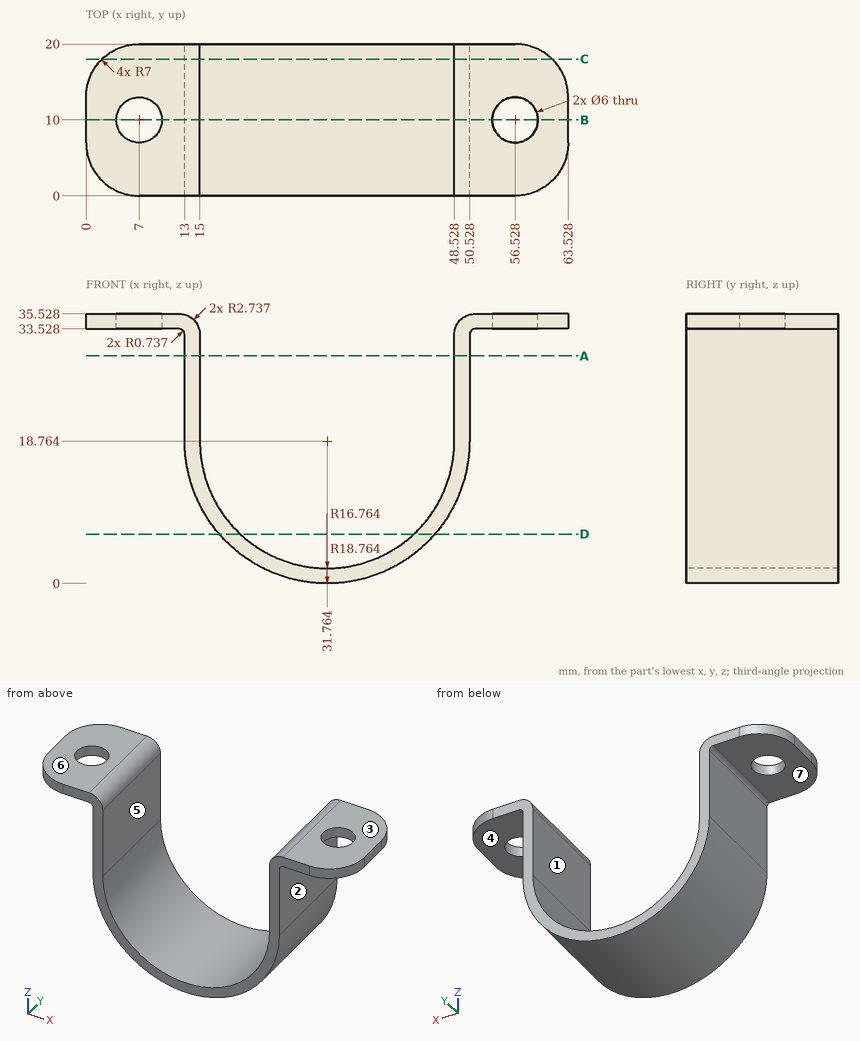
Part print with two shaded views. Sizes in mm from the minimum x, y, z corner. A direction names the side the tool comes from. Give positions to 0.01 mm unless a question says otherwise; leave off trailing zeros. Order: outer loops, then holes, each group sorted by start corner. A loop starts at its lowest first (then second) coordinate and runs counter-clockwise, first axis right, second up.
(1) Mould opens along X. For the marked faces 1, 2 and 3 say: released by +X, released by -X, zero draft, split by the parting line, or undercut.
(2) Saw through at A-A, the plane z = 30. Give the cut face in (x, y).
(3) Drill centre lines: L1, parallel to X at y = 8, z = 19; L2, parallel to Y at x = 7, z = 34; L3, parallel to X at y = 13.25, z = 16.5 (1 decimal). Where is each one in solid material? Low to high.
(4) Tool access for the marked faces 4, 5, 6 and 7: list every direction of +Z, -Z, +X, -X, +Y, -Y with a clear straight run to the whole face (end or side of a thin tool).
(5) Flat gauge pins, fed straight in: pin 1 (7 mm diameter, centred on y = 11, z = 24, fed in from -X); pin 2 (7 mm diameter, centred on y = 6, z = 27.5, fed in from +X); pin 3 (6 mm diameter, centred on x = 60.5, y = 7.5, fed in from -Z); pin 4 (5.5 mm diameter, centred on x = 7, y = 10, fed in from -Z). Where does each tip first touch, or does it go through?
(6) Saw through at C-C, the plane y = 18. Give the cut face in (x, z) (1 decimal).
(7) Saw through at D-D, the plane z = 6.5. Give the cut face in (x, y) (1 decimal).
(8) Saw through at B-B, the plane y = 10. Give the cut face in (x, z) (1 decimal).
Results found:
1. face 1: undercut
1. face 2: released by +X
1. face 3: zero draft
2. outline: (13, 0) - (15, 0) - (15, 20) - (13, 20) - close; (48.53, 0) - (50.53, 0) - (50.53, 20) - (48.53, 20) - close
3. L1: x = 13 to 15, 48.53 to 50.53
3. L2: y = 0 to 7, 13 to 20
3. L3: x = 13.1 to 15.2, 48.4 to 50.4
4. face 4: -Z, +X, +Y, -Y
4. face 5: +Z, +Y, -Y
4. face 6: +Z, +X, -X, +Y, -Y
4. face 7: -Z, -X, +Y, -Y
5. pin 1: stops at x = 13
5. pin 2: stops at x = 50.53
5. pin 3: stops at z = 33.53
5. pin 4: passes through
6. outline: (2.1, 33.5) - (12.3, 33.5) arc R0.7 cw to (13, 32.8) - (13, 18.8) arc R18.8 ccw to (50.5, 18.8) - (50.5, 32.8) arc R0.7 cw to (51.3, 33.5) - (61.4, 33.5) - (61.4, 35.5) - (51.3, 35.5) arc R2.7 ccw to (48.5, 32.8) - (48.5, 18.8) arc R16.8 cw to (15, 18.8) - (15, 32.8) arc R2.7 ccw to (12.3, 35.5) - (2.1, 35.5) - close
7. outline: (17.6, 0) - (20.3, 0) - (20.3, 20) - (17.6, 20) - close; (43.2, 0) - (46, 0) - (46, 20) - (43.2, 20) - close
8. outline: (0, 33.5) - (4, 33.5) - (4, 35.5) - (0, 35.5) - close; (10, 33.5) - (12.3, 33.5) arc R0.7 cw to (13, 32.8) - (13, 18.8) arc R18.8 ccw to (50.5, 18.8) - (50.5, 32.8) arc R0.7 cw to (51.3, 33.5) - (53.5, 33.5) - (53.5, 35.5) - (51.3, 35.5) arc R2.7 ccw to (48.5, 32.8) - (48.5, 18.8) arc R16.8 cw to (15, 18.8) - (15, 32.8) arc R2.7 ccw to (12.3, 35.5) - (10, 35.5) - close; (59.5, 33.5) - (63.5, 33.5) - (63.5, 35.5) - (59.5, 35.5) - close
